Geometry: final body of the model. Coordinates: model frame, mm. Give positions to 0.01 mm unless a question says otherwise; leave off trailing zeros. Loops run counter-clockwise (first coordinate to the right, second up) from the corner with the lowest first, then second, coordinate; pieces in that order, holes last.
1. First-contact query: P1, Ø1.5, axis at x = 0.5, y = -27.5, coming from the -Z side; P2, Ø4, axis at y = 0, z = 17.5, coming from the +X side. Flat tips, straight axial feed; report the tip coordinate or a pass-through.
2. Material intervals for line 1 along Y through (x, z) = (2.4, 19.5); line 2 along Y through (x, z) = (1.45, 11.5); line 3 along Y through (x, z) = (2.1, -17), sorted ascending.
3. Section B-B, the plane y = -10. Output: boundary loops of the cut face in (x, z).
4. Section C-C, the plane x = 1.75. State how many separate pieces and enclosed holes the cut face has, then the cut area to 3 significant figures.
5. Section A-A, the plane z = 28. Output: boundary loops of the cut face in (x, y), then the cut area to 3 significant figures.
6. Section D-D, the plane y = 24. Output: boundary loops of the cut face in (x, z).
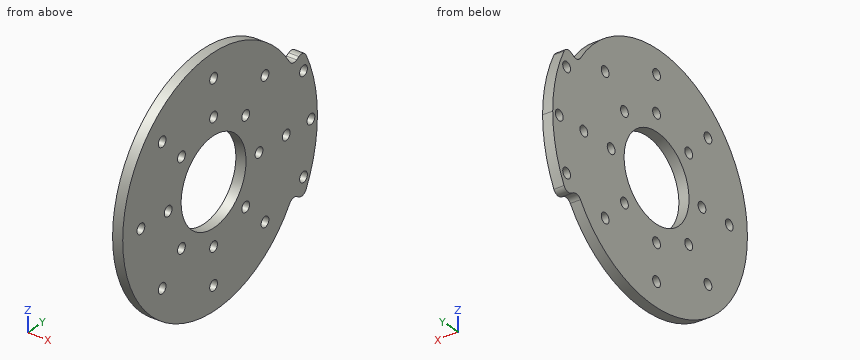
from build123d import *

# Parameters (mm, degrees)
SKETCH_1_R          = 35
EXTRUDE_1_DEPTH     = 3
SKETCH_2_R          = 1.5
CUT_EXTRUDE_1_DEPTH = 3
SKETCH_3_R          = 1.5
CUT_EXTRUDE_2_DEPTH = 3
SKETCH_4_R          = 12.5
CUT_EXTRUDE_3_DEPTH = 3
EXTRUDE_START       = -3
EXTRUDE_4_DEPTH     = 3
FILLET_1_R          = 2
FILLET_2_R          = 2
FILLET_3_R          = 2
FILLET_4_R          = 2
SKETCH_6_R          = 1.5
CUT_EXTRUDE_4_DEPTH = 3


with BuildPart() as part:
    # 草图1 → 凸台-拉伸1 (new body)
    with BuildSketch(Plane(origin=(0, 0, 0), x_dir=(0, 0, -1), z_dir=(1, 0, 0))):
        Circle(SKETCH_1_R)
    extrude(amount=EXTRUDE_1_DEPTH)

    # 草图2 → 切除-拉伸1 (cut)
    with BuildSketch(Plane(origin=(3, 0, 0), x_dir=(0, 0, -1), z_dir=(1, 0, 0))):
        with Locations((0, 28)):
            Circle(SKETCH_2_R)
        with Locations((19.798989873, 19.798989873)):
            Circle(SKETCH_2_R)
        with Locations((28, 0)):
            Circle(SKETCH_2_R)
        with Locations((19.798989873, -19.798989873)):
            Circle(SKETCH_2_R)
        with Locations((0, -28)):
            Circle(SKETCH_2_R)
        with Locations((-19.798989873, -19.798989873)):
            Circle(SKETCH_2_R)
        with Locations((-28, 0)):
            Circle(SKETCH_2_R)
        with Locations((-19.798989873, 19.798989873)):
            Circle(SKETCH_2_R)
    extrude(amount=-CUT_EXTRUDE_1_DEPTH, mode=Mode.SUBTRACT)

    # 草图3 → 切除-拉伸2 (cut)
    with BuildSketch(Plane(origin=(3, 0, 0), x_dir=(0, 0, -1), z_dir=(1, 0, 0))):
        with Locations((0, 17.5)):
            Circle(SKETCH_3_R)
        with Locations((12.374368671, 12.374368671)):
            Circle(SKETCH_3_R)
        with Locations((17.5, 0)):
            Circle(SKETCH_3_R)
        with Locations((12.374368671, -12.374368671)):
            Circle(SKETCH_3_R)
        with Locations((0, -17.5)):
            Circle(SKETCH_3_R)
        with Locations((-12.374368671, -12.374368671)):
            Circle(SKETCH_3_R)
        with Locations((-17.5, 0)):
            Circle(SKETCH_3_R)
        with Locations((-12.374368671, 12.374368671)):
            Circle(SKETCH_3_R)
    extrude(amount=-CUT_EXTRUDE_2_DEPTH, mode=Mode.SUBTRACT)

    # 草图4 → 切除-拉伸3 (cut)
    with BuildSketch(Plane.ZY):
        Circle(SKETCH_4_R)
    extrude(amount=-CUT_EXTRUDE_3_DEPTH, mode=Mode.SUBTRACT)

    # 草图5 → 凸台-拉伸4 (add)
    with BuildSketch(Plane(origin=(3, 0, 0), x_dir=(0, 0, -1), z_dir=(1, 0, 0)).offset(EXTRUDE_START)):
        with BuildLine():
            Line((-20, 34.641016151), (-17.5, 30.310889132))
            ThreePointArc((-17.5, 30.310889132), (-9.058666579, 33.80740392), (0, 35))
            Line((0, 35), (0, 40))
            ThreePointArc((0, 40), (-10.352761804, 38.637033052), (-20, 34.641016151))
        make_face()
        with BuildLine():
            ThreePointArc((0, 35), (9.058666579, 33.80740392), (17.5, 30.310889132))
            Line((17.5, 30.310889132), (20, 34.641016151))
            ThreePointArc((20, 34.641016151), (10.352761804, 38.637033052), (0, 40))
            Line((0, 40), (0, 35))
        make_face()
    extrude(amount=EXTRUDE_4_DEPTH)

    # 圆角1
    fillet_1_edges = [part.edges().sort_by_distance(p)[0] for p in [
        (1.5, 34.641016151, 20),
    ]]
    fillet(fillet_1_edges, radius=FILLET_1_R)

    # 圆角2
    fillet_2_edges = [part.edges().sort_by_distance(p)[0] for p in [
        (1.5, 30.310889132, 17.5),
    ]]
    fillet(fillet_2_edges, radius=FILLET_2_R)

    # 圆角3
    fillet_3_edges = [part.edges().sort_by_distance(p)[0] for p in [
        (1.5, 30.310889132, -17.5),
    ]]
    fillet(fillet_3_edges, radius=FILLET_3_R)

    # 圆角4
    fillet_4_edges = [part.edges().sort_by_distance(p)[0] for p in [
        (1.5, 34.641016151, -20),
    ]]
    fillet(fillet_4_edges, radius=FILLET_4_R)

    # 草图6 → 切除-拉伸4 (cut)
    with BuildSketch(Plane(origin=(3, 0, 0), x_dir=(0, 0, -1), z_dir=(1, 0, 0))):
        with Locations((0, 37.5)):
            Circle(SKETCH_6_R)
        with Locations((14.350628714, 34.645482469)):
            Circle(SKETCH_6_R)
        with Locations((-14.350628714, 34.645482469)):
            Circle(SKETCH_6_R)
    extrude(amount=-CUT_EXTRUDE_4_DEPTH, mode=Mode.SUBTRACT)


solid = part.part
Answers below:
1. P1: stops at z = -22.57
1. P2: stops at x = 3
2. line 1: y = -29.06 to -21.27, -18.33 to 18.33, 21.27 to 29.06
2. line 2: y = -33.06 to -13.59, -11.16 to -4.9, 4.9 to 11.16, 13.59 to 38.31
2. line 3: y = -30.59 to -1.41, 1.41 to 36.21
3. outline: (0, -33.54) - (3, -33.54) - (3, -7.5) - (0, -7.5) - close; (0, 7.5) - (3, 7.5) - (3, 33.54) - (0, 33.54) - close
4. separate pieces: 1
4. enclosed holes: 20
4. area: 3,420 mm2
5. outline: (0, -21) - (3, -21) - (3, -1.5) - (0, -1.5) - close; (0, 1.5) - (3, 1.5) - (3, 21) - (0, 21) - close
5. area: 117 mm2
6. outline: (0, -25.48) - (3, -25.48) - (3, 25.48) - (0, 25.48) - close
